Autodesk Inventor part; units mm, degrees
ref_plane "YZ Plane" through (0, 0, 0) normal (1, 0, 0) x (0, 1, 0)
ref_plane "XZ Plane" through (0, 0, 0) normal (0, 1, 0) x (-1, 0, 0)
ref_plane "XY Plane" through (0, 0, 0) normal (0, 0, 1) x (1, 0, 0)
sketch "Эскиз1" plane through (0, 0, 0) normal (0, 1, 0) x (-1, 0, 0)
  line L0 (-14, 14) -> (14, 14)
  line L1 (14, 14) -> (14, -14)
  line L2 (14, -14) -> (-14, -14)
  line L3 (-14, -14) -> (-14, 14)
  line L4 (-14, 14) -> (14, -14) construction
  line L5 (14, 14) -> (-14, -14) construction
  point P0 (0, 0)
  dimension "d0" = 28
  dimension "d1" = 28
extrude "Выдавливание1" add sketch "Эскиз1" along normal blind 56
sketch "Эскиз2" plane through (0, 0, 0) normal (0, -1, 0) x (1, 0, 0)
  circle A0 centre (0, 0) radius 4
extrude "Выдавливание2" cut sketch "Эскиз2" against normal blind 32
sketch "Эскиз3" plane through (-14, 0, -14) normal (-1, 0, 0) x (0, 0, 1)
  circle A0 centre (14, 46) radius 2
  point P0 (14, 0)
  dimension "d24" = 4
extrude "Выдавливание3" cut sketch "Эскиз3" against normal through all
sketch "Эскиз4" plane through (14, 0, 14) normal (1, 0, 0) x (0, 0, -1)
  circle A0 centre (14, 46) radius 2
  line L0 (9.6699, 46) -> (11.8349, 49.75)
  line L1 (11.8349, 49.75) -> (16.1651, 49.75)
  line L2 (16.1651, 49.75) -> (18.3301, 46)
  line L3 (18.3301, 46) -> (16.1651, 42.25)
  line L4 (16.1651, 42.25) -> (11.8349, 42.25)
  line L5 (11.8349, 42.25) -> (9.6699, 46)
  line L6 (0, 56) -> (28, 56)
  point P0 (14, 0)
  dimension "d8" = 7.5
extrude "Выдавливание4" cut sketch "Эскиз4" against normal blind 22
chamfer "Фаска1" distance 2 angle 45 6 edges at (14, 42.25, 0) (14, 44.125, -3.2476) (14, 47.875, -3.2476) (14, 49.75, 0) (14, 47.875, 3.2476) (14, 44.125, 3.2476)
ref_plane "РабПлоскость1" through (0, 22, 0) normal (0, -1, 0) x (1, 0, 0)
sketch "Эскиз5" plane through (0, 22, 0) normal (0, -1, 0) x (1, 0, 0)
  line L0 (0, 8.0829) -> (7, 4.0415)
  line L1 (7, 4.0415) -> (7, -4.0415)
  line L2 (7, -4.0415) -> (0, -8.0829)
  line L3 (0, -8.0829) -> (-7, -4.0415)
  line L4 (-7, -4.0415) -> (-7, 4.0415)
  line L5 (-7, 4.0415) -> (0, 8.0829)
  line L6 (0, 8.0829) -> (-14, 8.0829)
  line L7 (-14, -14) -> (-14, 14)
  line L8 (0, -8.0829) -> (-14, -8.0829)
  line L9 (-14, 8.0829) -> (-14, -8.0829)
  point P0 (0, 0)
  point P1 (0, 0)
  dimension "d15" = 14
extrude "Выдавливание5" cut sketch "Эскиз5" along normal mid plane 10
move faces "Перенос1" translate (2, 0, 0) faces at (-14, 5.6667, -2.6943)
sketch "Эскиз7" plane through (14, 0, 14) normal (0, 0, 1) x (1, 0, 0)
  line L0 (-10, 32) -> (-18, 32)
  line L1 (-2, 42.25) -> (-22, 42.25)
  circle A0 centre (-14, 37.125) radius 2
  line L2 (-14, 32) -> (-14, 42.25) construction
  point P0 (-14, 0)
  dimension "d28" = 4
extrude "Выдавливание7" cut sketch "Эскиз7" against normal blind 36.5
sketch "Эскиз8" plane through (14, 0, -14) normal (0, 0, -1) x (-1, 0, 0)
  circle A0 centre (14, 37.125) radius 2
  line L0 (18.3301, 37.125) -> (16.1651, 33.375)
  line L1 (16.1651, 33.375) -> (11.8349, 33.375)
  line L2 (11.8349, 33.375) -> (9.6699, 37.125)
  line L3 (9.6699, 37.125) -> (11.8349, 40.875)
  line L4 (11.8349, 40.875) -> (16.1651, 40.875)
  line L5 (16.1651, 40.875) -> (18.3301, 37.125)
  point P0 (14, 0)
  dimension "d31" = 7.5
extrude "Выдавливание8" cut sketch "Эскиз8" against normal blind 5
mirror "Зеркальное отражение1" about plane through (0, 0, 0) normal (0, 0, 1) of "Выдавливание8"
sketch "Эскиз10" plane through (14, 0, 14) normal (0, 0, 1) x (1, 0, 0)
  line L0 (0, 0) -> (0, 56)
  line L1 (-26, 0) -> (-26, 56)
  line L2 (0, 56) -> (-26, 56)
  line L3 (-26, 56) -> (-26, 32)
  line L4 (-26, 32) -> (0, 32)
  line L5 (0, 32) -> (0, 56)
  line L6 (-26, 0) -> (0, 0)
  point P0 (-14, 0)
  dimension "d35" = 32
equation "\"d1\" = d0"
equation "\"d2\" = 2 * d0"
properties part number "000.001.001 - Уголок" material "Пластик АБС"
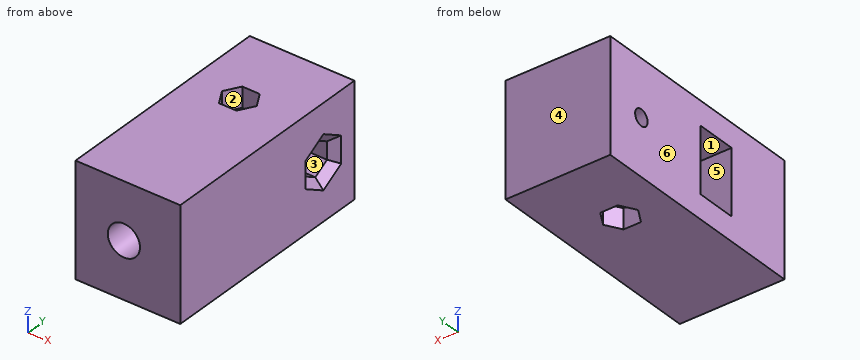
Read the model definition and answer for the solid it produces. Units are mm, in the model's axes. Face numbers are marked on the shaded views. A direction names the side the tool comes from. Round coordinates to 2 decimals unless told otherwise and drop trailing zeros. Loops run counter-clockwise (first coordinate to the right, second up) from the corner with the lowest first, then second, coordinate; pieces in that order, holes last.
Q1. Section C-C on y = 21.5 is taken. Write down the section's boundary in (x, z).
Q2. Determine the mould class of the marked faces 4, 5 and 6 for opening direction Y: released by +Y, released by -Y, zero draft, split by the parting line, or undercut.
Q3. Each of these flat-tipped pins is pushed along its axis until it touches: pin 1 (4.5 mm diameter, centred on x = 0, y = 37.125, fed in from -Z); pin 2 (4 mm diameter, centred on y = 45.5, z = -2, fed in from +X); pin 3 (3 mm diameter, centred on y = 19.5, z = 5, fed in from -X). Where does it stop, or does it pass through?
Q4. Which of the six approach directions +Z, -Z, +X, -X, +Y, -Y give full straight-line access (tool end or side, diameter ignored) to the marked faces 1, 2 and 3?
Q5. Section D-D on z = 5.75 is taken. Write down the section's boundary in (x, y) (3 decimals).
Q6. Section A-A on z = 0 is taken. Write down the section's boundary in (x, y) (3 decimals).
Q7. Consider probe 1 along Y at (x, z) = (0, -4.5) (3 decimals); probe 2 along Y at (x, z) = (0, -0.75) (3 decimals); probe 3 along Z at (x, y) = (7.5, 46.5). Determine where each line is inside the solid, lowest interval first.
Q8. Section B-B on x = 9 is taken. Write down the section's boundary in (y, z), and give its area (3 significant figures).
Output:
1. outline: (-12, -14) - (14, -14) - (14, 14) - (-12, 14) - (-12, 8.08) - (0, 8.08) - (7, 4.04) - (7, -4.04) - (0, -8.08) - (-12, -8.08) - close
2. face 4: released by +Y
2. face 5: undercut
2. face 6: zero draft
3. pin 1: stops at z = -9
3. pin 2: stops at x = 12.23
3. pin 3: stops at x = 2.74
4. face 1: -X
4. face 2: +Z
4. face 3: +X
5. outline: (-12, 0) - (14, 0) - (14, 44.459) - (13.23, 46) - (14, 47.541) - (14, 56) - (-12, 56) - (-12, 27) - (4.041, 27) - (4.041, 17) - (-12, 17) - close; hole circle Ø4 at (0, 37.125)
6. outline: (-12, 0) - (-4, 0) - (-4, 17) - (-12, 17) - close; (-12, 27) - (-4, 27) - (-4, 32) - (4, 32) - (4, 27) - (7, 27) - (7, 17) - (4, 17) - (4, 0) - (14, 0) - (14, 40.25) - (12, 42.25) - (-8, 42.25) - (-8, 44) - (-12, 44) - close; (-12, 48) - (-8, 48) - (-8, 49.75) - (12, 49.75) - (14, 51.75) - (14, 56) - (-12, 56) - close; hole circle Ø4 at (0, 37.125)
7. probe 1: y = 0 to 17, 27 to 35.125, 39.125 to 56
7. probe 2: y = 32 to 35.125, 39.125 to 42.25, 49.75 to 56
7. probe 3: z = -14 to -4.04, 4.04 to 14
8. outline: (0, -14) - (56, -14) - (56, 14) - (0, 14) - close; hole (42.25, -2.17) - (46, -4.33) - (49.75, -2.17) - (49.75, 2.17) - (46, 4.33) - (42.25, 2.17) - close
8. area: 1,520 mm2
